Geometry check sheet. Reference: the model listing, model coordinates, mm. Give positions to 0.01 mm unless a question says otherwise; leave off trailing zeros. Write each loop counter-clockwise with the first axis right and the second up, starting at its lowest first coordinate (ties: lowest second). Pieces come first, ordered by that corner, then holes. Notation, with made-up numbers: M -25.5,-30.5 L 21.5,-30.5 A7 ccw 21.5,-18.5 Z; hole C 54,27 d7. An arc over 180 degrees is marked long. One line per item, written item: value. Start each with the question number.
1. Cross-section at C-C on x = 36.5. Record the cut outline in (y, z), then the cut area to 3 significant figures.
2. Scan lines: line 1 (X direction, y = -1.15, z = 9.25); line 2 (X direction, y = -0.6, z = 1.5); line 3 (Z direction, x = 32, y = -0.85). Record each from-to range of solid material in increasing order.
3. Cross-section at A-A on z = 2. Record the cut outline in (x, y), then the cut area to 4 significant figures.
4. Cross-section at B-B on x = 18. Record the cut outline in (y, z).
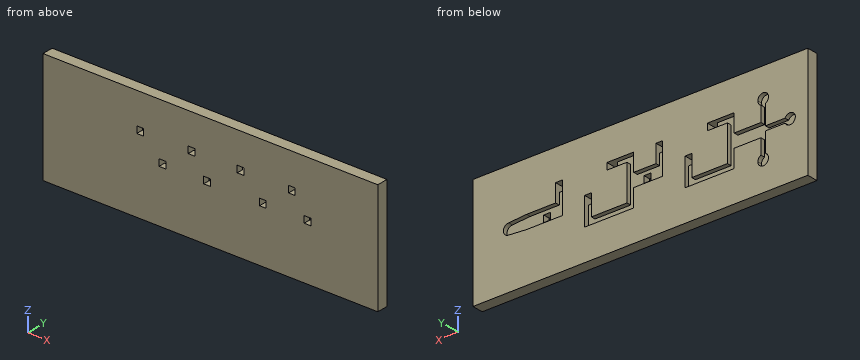
from build123d import *

# Parameters (mm, degrees)
SKETCH2_W           = 75
SKETCH2_H           = 25
BOSS_EXTRUDE1_DEPTH = 2.5
CUT_EXTRUDE1_DEPTH  = 1
SKETCH3_W           = 1.5
SKETCH3_H           = 1.5
CUT_EXTRUDE2_DEPTH  = 3.5
SKETCH4_W           = 0.5
SKETCH4_H           = 1
CUT_EXTRUDE3_DEPTH  = 1


with BuildPart() as part:
    # Sketch2 → Boss-Extrude1 (new body)
    with BuildSketch(Plane(origin=(0, 0, 0), x_dir=(1, 0, 0), z_dir=(0, 1, 0))):
        with Locations((8.414308894, -4.186562074)):
            Rectangle(SKETCH2_W, SKETCH2_H)
    extrude(amount=-BOSS_EXTRUDE1_DEPTH)

    # Sketch1 → Cut-Extrude1 (cut)
    with BuildSketch(Plane(origin=(0, 0, 0), x_dir=(1, 0, 0), z_dir=(0, 1, 0))):
        Polygon((-12.585691106, -2.686562074), (-19.085691106, -2.686562074), (-19.085691106, -5.686562074), (-12.585691106, -5.686562074), (-12.585691106, -9.686562074), (-6.585691106, -9.686562074), (-6.585691106, -8.186562074), (-11.085691106, -8.186562074), (-11.085691106, -0.186562074), (-3.085691106, -0.186562074), (-3.085691106, -4.936562074), (-1.585691106, -4.936562074), (-1.585691106, 1.313437926), (-12.585691106, 1.313437926), align=None)
        Polygon((9.914308894, -2.686562074), (3.414308894, -2.686562074), (3.414308894, -9.686562074), (4.914308894, -9.686562074), (4.914308894, -5.686562074), (9.914308894, -5.686562074), (9.914308894, -9.686562074), (15.914308894, -9.686562074), (15.914308894, -8.186562074), (11.414308894, -8.186562074), (11.414308894, -0.186562074), (19.414308894, -0.186562074), (19.414308894, -4.936562074), (20.914308894, -4.936562074), (20.914308894, 1.313437926), (9.914308894, 1.313437926), align=None)
        Polygon((33.914308894, -2.686562074), (25.914308894, -2.686562074), (25.914308894, -9.686562074), (27.414308894, -9.686562074), (27.414308894, -5.686562074), (33.914308894, -5.686562074), align=None)
    extrude(amount=-CUT_EXTRUDE1_DEPTH, mode=Mode.SUBTRACT)

    # Sketch3 → Cut-Extrude2 (cut, through all)
    with BuildSketch(Plane(origin=(0, 0, 0), x_dir=(1, 0, 0), z_dir=(0, 1, 0))):
        with Locations((-7.335691106, -8.936562074)):
            Rectangle(SKETCH3_W, SKETCH3_H)
        with Locations((-2.335691106, -4.186562074)):
            Rectangle(SKETCH3_W, SKETCH3_H)
        with Locations((4.164308894, -8.936562074)):
            Rectangle(SKETCH3_W, SKETCH3_H)
        with Locations((30.164308894, -4.186562074)):
            Rectangle(SKETCH3_W, SKETCH3_H)
        with Locations((7.664308894, -4.186562074)):
            Rectangle(SKETCH3_W, SKETCH3_H)
        with Locations((15.164308894, -8.936562074)):
            Rectangle(SKETCH3_W, SKETCH3_H)
        with Locations((20.164308894, -4.186562074)):
            Rectangle(SKETCH3_W, SKETCH3_H)
        with Locations((26.664308894, -8.936562074)):
            Rectangle(SKETCH3_W, SKETCH3_H)
    extrude(amount=-CUT_EXTRUDE2_DEPTH, mode=Mode.SUBTRACT)

    # Sketch4 → Cut-Extrude3 (cut)
    with BuildSketch(Plane(origin=(0, 0, 0), x_dir=(1, 0, 0), z_dir=(0, 1, 0))):
        with BuildLine():
            ThreePointArc((37.914308894, -5.386562074), (39.114308894, -4.186562074), (37.914308894, -2.986562074))
            Line((37.914308894, -2.986562074), (33.914308894, -2.686562074))
            Line((33.914308894, -2.686562074), (33.914308894, -5.686562074))
            Line((33.914308894, -5.686562074), (37.914308894, -5.386562074))
        make_face()
        with BuildLine():
            ThreePointArc((-17.885691106, 1.813437926), (-19.733765176, 2.82338842), (-19.585691106, 0.722566715))
            Line((-19.585691106, 0.722566715), (-19.585691106, 1.813437926))
            ThreePointArc((-19.585691106, 1.813437926), (-19.085691106, 2.313437926), (-18.585691106, 1.813437926))
            Line((-18.585691106, 1.813437926), (-18.585691106, 0.722566715))
            ThreePointArc((-18.585691106, 0.722566715), (-18.075740612, 1.165363856), (-17.885691106, 1.813437926))
        make_face()
        with BuildLine():
            Line((-19.585691106, 1.813437926), (-19.585691106, 0.722566715))
            ThreePointArc((-19.585691106, 0.722566715), (-19.085691106, 0.613437926), (-18.585691106, 0.722566715))
            Line((-18.585691106, 0.722566715), (-18.585691106, 1.813437926))
            ThreePointArc((-18.585691106, 1.813437926), (-19.085691106, 2.313437926), (-19.585691106, 1.813437926))
        make_face()
        with BuildLine():
            Line((-19.585691106, 0.722566715), (-19.585691106, -3.686562074))
            Line((-19.585691106, -3.686562074), (-19.085691106, -3.686562074))
            Line((-19.085691106, -3.686562074), (-19.085691106, -2.686562074))
            Line((-19.085691106, -2.686562074), (-18.585691106, -2.686562074))
            Line((-18.585691106, -2.686562074), (-18.585691106, 0.722566715))
            ThreePointArc((-18.585691106, 0.722566715), (-19.085691106, 0.613437926), (-19.585691106, 0.722566715))
        make_face()
        with BuildLine():
            Line((-23.994819895, -4.686562074), (-25.085691106, -4.686562074))
            ThreePointArc((-25.085691106, -4.686562074), (-25.585691106, -4.186562074), (-25.085691106, -3.686562074))
            Line((-25.085691106, -3.686562074), (-23.994819895, -3.686562074))
            ThreePointArc((-23.994819895, -3.686562074), (-26.285691106, -4.186562074), (-23.994819895, -4.686562074))
        make_face()
        with BuildLine():
            ThreePointArc((-25.085691106, -3.686562074), (-25.585691106, -4.186562074), (-25.085691106, -4.686562074))
            Line((-25.085691106, -4.686562074), (-23.994819895, -4.686562074))
            ThreePointArc((-23.994819895, -4.686562074), (-23.913290694, -4.442447347), (-23.885691106, -4.186562074))
            ThreePointArc((-23.885691106, -4.186562074), (-23.913290694, -3.9306768), (-23.994819895, -3.686562074))
            Line((-23.994819895, -3.686562074), (-25.085691106, -3.686562074))
        make_face()
        with BuildLine():
            ThreePointArc((-23.885691106, -4.186562074), (-23.913290694, -4.442447347), (-23.994819895, -4.686562074))
            Line((-23.994819895, -4.686562074), (-19.585691106, -4.686562074))
            Line((-19.585691106, -4.686562074), (-19.585691106, -3.686562074))
            Line((-19.585691106, -3.686562074), (-23.994819895, -3.686562074))
            ThreePointArc((-23.994819895, -3.686562074), (-23.913290694, -3.9306768), (-23.885691106, -4.186562074))
        make_face()
        with Locations((-19.335691106, -4.186562074)):
            Rectangle(SKETCH4_W, SKETCH4_H)
        with BuildLine():
            Line((-19.085691106, -3.686562074), (-19.085691106, -4.686562074))
            ThreePointArc((-19.085691106, -4.686562074), (-18.732137716, -4.540115464), (-18.585691106, -4.186562074))
            ThreePointArc((-18.585691106, -4.186562074), (-18.732137716, -3.833008683), (-19.085691106, -3.686562074))
        make_face()
        with BuildLine():
            ThreePointArc((-19.085691106, -3.686562074), (-18.732137716, -3.833008683), (-18.585691106, -4.186562074))
            Line((-18.585691106, -4.186562074), (-18.585691106, -2.686562074))
            Line((-18.585691106, -2.686562074), (-19.085691106, -2.686562074))
            Line((-19.085691106, -2.686562074), (-19.085691106, -3.686562074))
        make_face()
        with BuildLine():
            Line((-19.585691106, -10.186562074), (-19.585691106, -9.095690862))
            ThreePointArc((-19.585691106, -9.095690862), (-19.733765176, -11.196512568), (-17.885691106, -10.186562074))
            ThreePointArc((-17.885691106, -10.186562074), (-18.075740612, -9.538488004), (-18.585691106, -9.095690862))
            Line((-18.585691106, -9.095690862), (-18.585691106, -10.186562074))
            ThreePointArc((-18.585691106, -10.186562074), (-19.085691106, -10.686562074), (-19.585691106, -10.186562074))
        make_face()
        with BuildLine():
            ThreePointArc((-18.585691106, -9.095690862), (-19.085691106, -8.986562074), (-19.585691106, -9.095690862))
            Line((-19.585691106, -9.095690862), (-19.585691106, -10.186562074))
            ThreePointArc((-19.585691106, -10.186562074), (-19.085691106, -10.686562074), (-18.585691106, -10.186562074))
            Line((-18.585691106, -10.186562074), (-18.585691106, -9.095690862))
        make_face()
        with BuildLine():
            Line((-19.085691106, -4.686562074), (-19.585691106, -4.686562074))
            Line((-19.585691106, -4.686562074), (-19.585691106, -9.095690862))
            ThreePointArc((-19.585691106, -9.095690862), (-19.085691106, -8.986562074), (-18.585691106, -9.095690862))
            Line((-18.585691106, -9.095690862), (-18.585691106, -5.686562074))
            Line((-18.585691106, -5.686562074), (-19.085691106, -5.686562074))
            Line((-19.085691106, -5.686562074), (-19.085691106, -4.686562074))
        make_face()
        with BuildLine():
            ThreePointArc((-18.585691106, -4.186562074), (-18.732137716, -4.540115464), (-19.085691106, -4.686562074))
            Line((-19.085691106, -4.686562074), (-19.085691106, -5.686562074))
            Line((-19.085691106, -5.686562074), (-18.585691106, -5.686562074))
            Line((-18.585691106, -5.686562074), (-18.585691106, -4.186562074))
        make_face()
    extrude(amount=-CUT_EXTRUDE3_DEPTH, mode=Mode.SUBTRACT)


solid = part.part
Report:
1. outline: M -2.5,-8.31 L 0,-8.31 L 0,2.88 L -1,2.88 L -1,5.49 L 0,5.49 L 0,16.69 L -2.5,16.69 Z
1. area: 59.9 mm^2
2. line 1: x = -29.09 to -8.09, -6.59 to 3.41, 4.91 to 14.41, 15.91 to 25.91, 27.41 to 45.91
2. line 2: x = -29.09 to -19.59, -18.59 to -12.59, -11.09 to -3.09, -1.59 to 9.91, 11.41 to 19.41, 20.91 to 45.91
2. line 3: z = -8.31 to 2.69, 5.69 to 16.69
3. outline: M -29.09,-2.5 L 45.91,-2.5 L 45.91,0 L 20.91,0 L 20.91,-1 L 19.41,-1 L 19.41,0 L 11.41,0 L 11.41,-1 L 9.91,-1 L 9.91,0 L -1.59,0 L -1.59,-1 L -3.09,-1 L -3.09,0 L -11.09,0 L -11.09,-1 L -12.59,-1 L -12.59,0 L -18.59,0 L -18.59,-1 L -19.59,-1 L -19.59,0 L -29.09,0 Z
3. area: 180.5 mm^2
4. outline: M -2.5,-8.31 L 0,-8.31 L 0,-1.31 L -1,-1.31 L -1,0.19 L 0,0.19 L 0,16.69 L -2.5,16.69 Z
